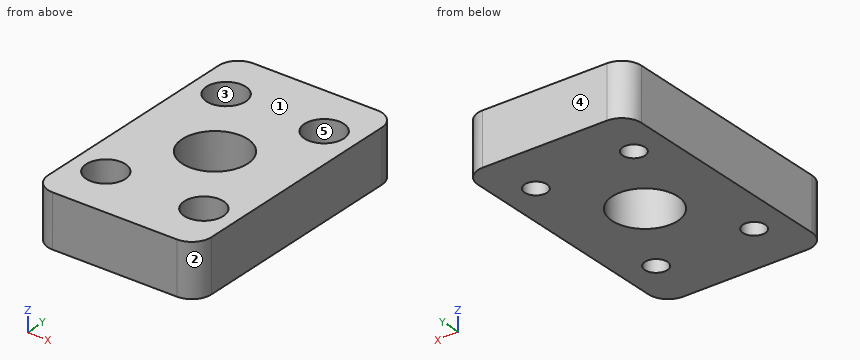
Autodesk Inventor part; units mm, degrees
ref_plane "YZ Plane" through (0, 0, 0) normal (1, 0, 0) x (0, 1, 0)
ref_plane "XZ Plane" through (0, 0, 0) normal (0, 1, 0) x (-1, 0, 0)
ref_plane "XY Plane" through (0, 0, 0) normal (0, 0, 1) x (1, 0, 0)
sketch "Skizze2" plane through (0, 0, 0) normal (0, 0, 1) x (1, 0, 0)
  line L0 (-9.5, -20) -> (9.5, -20)
  line L1 (12.5, -17) -> (12.5, 17)
  line L2 (9.5, 20) -> (-9.5, 20)
  line L3 (-12.5, 17) -> (-12.5, -17)
  line L4 (-12.5, -20) -> (12.5, 20) construction
  line L5 (12.5, -20) -> (-12.5, 20) construction
  circle A0 centre (0, 0) radius 5
  circle A1 centre (7.5, -12) radius 1.7
  circle A2 centre (-7.5, -12) radius 1.7
  circle A3 centre (7.5, 12) radius 1.7
  circle A4 centre (-7.5, 12) radius 1.7
  circle A5 centre (-7.5, 12) radius 3
  circle A6 centre (7.5, 12) radius 3
  circle A7 centre (7.5, -12) radius 3
  circle A8 centre (-7.5, -12) radius 3
  arc A9 (-12.5, -17) -> (-9.5, -20) centre (-9.5, -17) ccw
  arc A10 (9.5, -20) -> (12.5, -17) centre (9.5, -17) ccw
  arc A11 (12.5, 17) -> (9.5, 20) centre (9.5, 17) ccw
  arc A12 (-9.5, 20) -> (-12.5, 17) centre (-9.5, 17) ccw
  dimension "d0" = 40
  dimension "d1" = 25
  dimension "d9" = 10
  dimension "d11" = 3.4
  dimension "d12" = 3.4
  dimension "d13" = 3.4
  dimension "d14" = 3.4
  dimension "d15" = 15
  dimension "d16" = 24
  dimension "d17" = 6
  dimension "d18" = 6
  dimension "d19" = 6
  dimension "d20" = 6
  dimension "d21" = 3
extrude "Extrusion1" add sketch "Skizze2" along normal blind 8 contours A9 L3 A12 L2 A11 L1 A10 L0 | A0
extrude "Extrusion3" add sketch "Skizze2" along normal blind 4.6 contours A5 | A6 | A7 | A8
extrude "Extrusion4" cut sketch "Skizze2" along normal through all contours A0
properties part number "Adapterplatte_Focus"
Can you work these out from the model? Positions are in its coordinate system, mm. Face numbers are marked on the shaded views. A direction names the side the tool comes from. Round coordinates to 2 decimals unless told otherwise and drop trailing zeros. Order: outer loops, then holes, each group sorted by start corner. A loop starts at its lowest first (then second) coordinate and runs counter-clockwise, first axis right, second up. Notation, with made-up numbers: (83, -10.75) -> (114, -10.75) arc R27 cw to (114, 28.25) -> close; hole circle Ø2 at (49, -19.75). An arc over 180 degrees is marked (long way). Return JSON: item names as keys, results as strings. Group by question number.
1. We'd pull the mould along Y, two halves only. Please class the marked faces 1, 2 and 3: released by +Y, released by -Y, zero draft, split by the parting line, or undercut.
2. If we section it at B-B, the plane x = -7.5: Write out the boundary of the cut face in (y, z).
3. If we section it at D-D, the plane z = 3: Write out the boundary of the cut face in (x, y), then the cut area to 3 significant figures.
4. Which directions (+Z, -Z, +X, -X, +Y, -Y) give clear straight access to the entire face, cutting with the end or side of a thin tool? Please do the marked faces 4 and 5.
5. I need wall thicknesses on line 1 (Y direction, x = 7.5, z = 5.6); line 2 (Y direction, x = 7.5, z = 2.3); line 3 (Y direction, x = 0, z = 6.25). Which ranges of each line are inside material? Lowest first, please. Write a range as [from, to].
6. If we section it at A-A, the plane y = -12: Write out the boundary of the cut face in (x, z).
7. Will this pin go through, and if not, where does the flat tip stop? pin 1 (1.8 mm diameter, centred on x = -8.5, y = -13, fed in from +Z).
8. If we section it at C-C, the plane y = 0: Write out the boundary of the cut face in (x, z).
Output values:
{
 "1": {"face 1": "zero draft", "face 2": "released by -Y", "face 3": "undercut"},
 "2": {"outline": "(-20, 0) -> (-13.7, 0) -> (-13.7, 4.6) -> (-15, 4.6) -> (-15, 8) -> (-20, 8) -> close; (-10.3, 0) -> (10.3, 0) -> (10.3, 4.6) -> (9, 4.6) -> (9, 8) -> (-9, 8) -> (-9, 4.6) -> (-10.3, 4.6) -> close; (13.7, 0) -> (20, 0) -> (20, 8) -> (15, 8) -> (15, 4.6) -> (13.7, 4.6) -> close"},
 "3": {"outline": "(-12.5, -17) arc R3 ccw to (-9.5, -20) -> (9.5, -20) arc R3 ccw to (12.5, -17) -> (12.5, 17) arc R3 ccw to (9.5, 20) -> (-9.5, 20) arc R3 ccw to (-12.5, 17) -> close; hole circle Ø3.4 at (-7.5, -12); hole circle Ø3.4 at (-7.5, 12); hole circle Ø10 at (0, 0); hole circle Ø3.4 at (7.5, -12); hole circle Ø3.4 at (7.5, 12)", "area": "877 mm²"},
 "4": {"face 4": "+Z, -Z, +X, -X, +Y", "face 5": "+Z"},
 "5": {"line 1": "[-20, -15], [-9, 9], [15, 20]", "line 2": "[-20, -13.7], [-10.3, 10.3], [13.7, 20]", "line 3": "[-20, -5], [5, 20]"},
 "6": {"outline": "(-12.5, 0) -> (-9.2, 0) -> (-9.2, 4.6) -> (-10.5, 4.6) -> (-10.5, 8) -> (-12.5, 8) -> close; (-5.8, 0) -> (5.8, 0) -> (5.8, 4.6) -> (4.5, 4.6) -> (4.5, 8) -> (-4.5, 8) -> (-4.5, 4.6) -> (-5.8, 4.6) -> close; (9.2, 0) -> (12.5, 0) -> (12.5, 8) -> (10.5, 8) -> (10.5, 4.6) -> (9.2, 4.6) -> close"},
 "7": {"pin 1": "z = 4.6"},
 "8": {"outline": "(-12.5, 0) -> (-5, 0) -> (-5, 8) -> (-12.5, 8) -> close; (5, 0) -> (12.5, 0) -> (12.5, 8) -> (5, 8) -> close"}
}
